Input: part model. Units: mm. Frame: model coordinates. A direction names the side the tool comes from. Give positions to 0.01 mm unless a question says otherwise; leave off trailing zeros. Answer in a Markdown table with one row per item. Add a question column.
from build123d import *

# Parameters (mm, degrees)
BOSS_EXTRUDE1_DEPTH = 6.35
SKETCH3_W           = 4
SKETCH3_H           = 12
CUT_EXTRUDE1_DEPTH  = 6.35
SKETCH4_R           = 1.55
CUT_EXTRUDE2_DEPTH  = 7.35
SKETCH5_R           = 1.55
CUT_EXTRUDE3_DEPTH  = 7.35


with BuildPart() as part:
    # Sketch2 → Boss-Extrude1 (new body)
    with BuildSketch(Plane.XY):
        with BuildLine():
            Line((77.5, 93.15), (-77.5, 93.15))
            ThreePointArc((-77.5, 93.15), (-84.217514421, 90.367514421), (-87, 83.65))
            Line((-87, 83.65), (-87, -83.65))
            ThreePointArc((-87, -83.65), (-84.217514421, -90.367514421), (-77.5, -93.15))
            Line((-77.5, -93.15), (77.5, -93.15))
            ThreePointArc((77.5, -93.15), (83.579939001, -90.037313843), (86, -83.65))
            Line((86, -83.65), (86, 83.65))
            ThreePointArc((86, 83.65), (83.579939001, 90.037313843), (77.5, 93.15))
        make_face()
    extrude(amount=BOSS_EXTRUDE1_DEPTH)

    # Sketch3 → Cut-Extrude1 (cut)
    with BuildSketch(Plane.XY.offset(6.35)):
        with Locations((79, 6)):
            Rectangle(SKETCH3_W, SKETCH3_H)
    extrude(amount=-CUT_EXTRUDE1_DEPTH, mode=Mode.SUBTRACT)

    # Sketch4 → Cut-Extrude2 (cut, through all)
    with BuildSketch(Plane.XY.offset(6.35)):
        with Locations((-68.2, 71.8)):
            Circle(SKETCH4_R)
        with Locations((-68.2, 57.8)):
            Circle(SKETCH4_R)
        with Locations((-68.2, -57.8)):
            Circle(SKETCH4_R)
        with Locations((-68.2, -71.8)):
            Circle(SKETCH4_R)
    extrude(amount=-CUT_EXTRUDE2_DEPTH, mode=Mode.SUBTRACT)

    # Sketch5 → Cut-Extrude3 (cut, through all)
    with BuildSketch(Plane.XY.offset(6.35)):
        with Locations((79, 16.45)):
            Circle(SKETCH5_R)
        with Locations((79, -9.55)):
            Circle(SKETCH5_R)
    extrude(amount=-CUT_EXTRUDE3_DEPTH, mode=Mode.SUBTRACT)


solid = part.part
Q1. Contact query for flat-ended pins moving along their axis: P1, Ø3.5, axis at x = -68.2, y = 71.8, coming from the +Z side; P2, Ø2, axis at x = 79, z = 3.5, coming from the +Y side; P3, Ø3, axis at x = -68.2, y = -71.8, coming from the +Z side. Output: stop coordinate, or through.
Q2. Line query: probe 1 along Y at (x, z) = (-68.2, 1.5); probe 2 along X at (y, z) = (10.5, 4.75); probe 3 along X at (y, z) = (-58.5, 4.25). Output: solid intervals per line, ascending.
Q3. Access query for faces 5 (the flat face through (-2, 1, 0)), 6 (the flat face through (79, 12, 3)). Directions: +Z, -Z, +X, -X, +Y, -Y. A direction counts if a zero-diameter tool reaches every point of the face in a straight line with its end or side. Return the directions, or none.
Q4. Pull-direction query (Y, two-part tool) for faces 1 (the flat face through (-2, 1, 6.35)), 2 (the flat face through (79, 0, 3)), 3 (the cylindrical face through (-84.143, 90.441, 3.131)), 4 (the cylindrical face through (-84.291, -90.293, 3.131)); classes: +Y half, -Y half, draft (parallel to the pull), parting line (faces both ways), or undercut.
Computed:
| question | item | result |
|---|---|---|
| 1 | P1 | stops at z = 6.35 |
| 1 | P2 | stops at y = 93.08 |
| 1 | P3 | passes through |
| 2 | probe 1 | y = -93.15 to -73.35, -70.25 to -59.35, -56.25 to 56.25, 59.35 to 70.25, 73.35 to 93.15 |
| 2 | probe 2 | x = -87 to 77, 81 to 86 |
| 2 | probe 3 | x = -87 to -69.58, -66.82 to 86 |
| 3 | face 5 | -Z, +X, -X, +Y, -Y |
| 3 | face 6 | +Z, -Z |
| 4 | face 1 | draft |
| 4 | face 2 | undercut |
| 4 | face 3 | +Y half |
| 4 | face 4 | -Y half |
